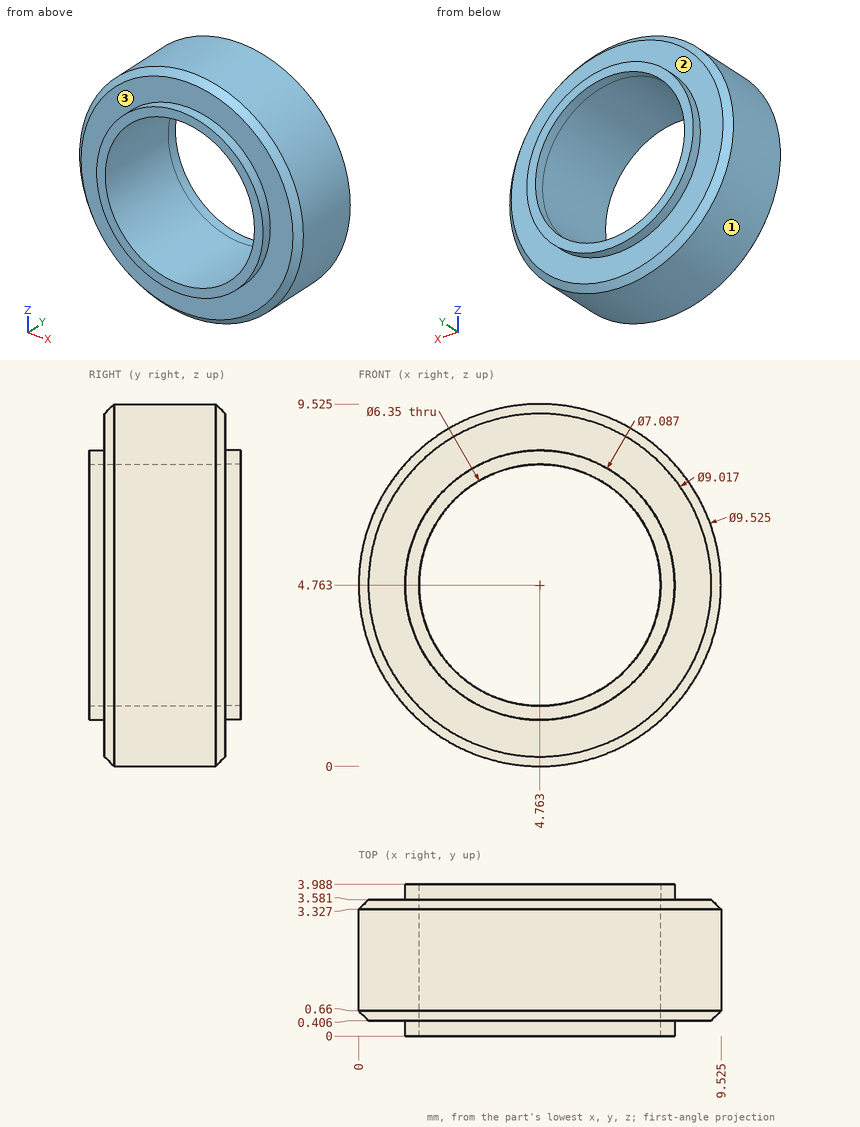
Part print with two shaded views. Sizes in mm from the minimum x, y, z corner. A direction names the side the tool comes from. Coordinates: 2 decimals unless noted, no trailing zeros. Answer in a Markdown table with one row per item.
1. Flat gauge pins, fed straight in: P1, Ø1, axis at x = 7, y = 3.5, coming from the +Z side (1 decimal); P2, Ø3, axis at x = 7, z = 7.5, coming from the -Y side; P3, Ø2, axis at x = 6.5, y = 1.5, coming from the -Z side. Where does each tip first touch, or does it go through?
Answer:
| item | result |
|---|---|
| P1 | z = 9.2 |
| P2 | y = 0 |
| P3 | z = 0.06 |
2. 3-axis set-ups, long thin cutter, end or side, ignore diameter. For the marked faces 1, 2 and 3: which of +Z, -Z, +X, -X, +Y, -Y reach the whole face in a straight line?
Answer:
| item | result |
|---|---|
| face 1 | +Y, -Y |
| face 2 | +Y |
| face 3 | -Y |
3. Drill centre lines: L1, parallel to Y at x = 1.25, z = 5.75; L2, parallel to X at y = 0.9, z = 5.75 (1 decimal); L3, parallel to X at y = 0.25, z = 4.25 (1 decimal). Where is each one in solid material? Low to high. Write a range as from..to.
Answer:
| item | result |
|---|---|
| L1 | 0.41..3.58 |
| L2 | 0.1..1.7, 7.8..9.4 |
| L3 | 1.3..1.6, 7.9..8.3 |
